The listing builds one solid part. Answer for the finished solid, in the listing's coordinates (mm). Give positions to 0.01 mm unless a question says otherwise; leave off trailing zeros. Loops run counter-clockwise (first coordinate to the right, second up) from the corner with the lowest first, then second, coordinate; pieces in that order, holes last. Notation, with made-up numbers: M -26,-33 L 15,-33 A15 cw 15,-16 Z; hole C 35,38 d7. An arc over 180 degrees is marked long. One line per item, written item: value. Start each with the question number.
Q1. A cutting plane is placed at C-C, the plane z = 36. Determine the outline of the cut face in (x, y).
Q2. A cutting plane is placed at B-B, the plane y = -5. Determine the outline of the cut face in (x, z), and give its area (3 significant figures).
Q3. A cutting plane is placed at D-D, the plane y = 39.5. Determine the outline of the cut face in (x, z).
Q4. Consider L1, parallel to Y at x = 1.3, z = 9; L2, parallel to Y at x = 0.4, z = 4; L3, parallel to Z at x = -2.15, y = 33. Determine where each line is inside the solid, lowest interval first.
Q5. A cutting plane is placed at A-A, the plane z = 4. Determine the outline of the cut face in (x, y).
from build123d import *

# Parameters (mm, degrees)
SKETCH1_R                = 59
EXTRUDE1_DEPTH           = 3
EXTRUDE2_DEPTH           = 3
CIRPATTERN1_COUNT        = 6
F_2_0_2_DIAMETER_HOLE1_D = 2
F_2_0_2_DIAMETER_HOLE3_D = 2
F_2_0_2_DIAMETER_HOLE4_D = 2
CIRPATTERN2_COUNT        = 6
CIRPATTERN3_COUNT        = 4
CIRPATTERN3_ANGLE        = 180


with BuildPart() as part:
    # Sketch1 → Extrude1 (new, symmetric)
    with BuildSketch(Plane(origin=(0, 0, 0), x_dir=(0, 0, -1), z_dir=(1, 0, 0))):
        Circle(SKETCH1_R)
        Polygon((27.939644545, 7.486405193), (7.486405193, 27.939644545), (-20.453239352, 20.453239352), (-27.939644545, -7.486405193), (-7.486405193, -27.939644545), (20.453239352, -20.453239352), align=None, mode=Mode.SUBTRACT)
    extrude(amount=EXTRUDE1_DEPTH, both=True)

    # Sketch2 → Extrude2 (add, symmetric)
    with BuildSketch(Plane(origin=(0, 0, 0), x_dir=(0, 0, -1), z_dir=(1, 0, 0))):
        with BuildLine():
            Line((-2, 67.961805723), (-0.262709442, 61.478149092))
            ThreePointArc((-0.262709442, 61.478149092), (-0.58620663, 59.77173183), (-2.122608272, 58.961805723))
            ThreePointArc((-2.122608272, 58.961805723), (28.679663449, 51.560419941), (51.21368579, 29.294340542))
            ThreePointArc((51.21368579, 29.294340542), (36.791707484, 48.186627241), (17.927108603, 62.644803614))
            ThreePointArc((17.927108603, 62.644803614), (8.312130826, 66.609702921), (-2, 67.961805723))
        make_face()
    extrude2 = extrude(amount=EXTRUDE2_DEPTH, both=True)

    # CirPattern1: Extrude2 ×6 about axis
    cirpattern1_axis = Axis((0, 0, 0), (1, 0, 0))
    for i in range(1, CIRPATTERN1_COUNT):
        add(extrude2.rotate(cirpattern1_axis, i * 360 / CIRPATTERN1_COUNT))

    # Ø2.0 (2) Diameter Hole1 (through all)
    with Locations(Plane(origin=(3, 0, 0), x_dir=(0, 0, -1), z_dir=(1, 0, 0))):
        with Locations((7.486405193, 27.939644545), (27.939644545, 7.486405193), (20.453239352, -20.453239352), (-7.486405193, -27.939644545), (-27.939644545, -7.486405193), (-20.453239352, 20.453239352)):
            Hole(F_2_0_2_DIAMETER_HOLE1_D / 2)

    # Ø2.0 (2) Diameter Hole3 (through all)
    with Locations(Plane(origin=(3, 0, 0), x_dir=(0, 0, -1), z_dir=(1, 0, 0))):
        with Locations((14.539853904, 20.886195834)):
            f_2_0_2_diameter_hole3 = Hole(F_2_0_2_DIAMETER_HOLE3_D / 2)

    # Ø2.0 (2) Diameter Hole4 (through all)
    with Locations(Plane(origin=(3, 0, 0), x_dir=(0, 0, -1), z_dir=(1, 0, 0))):
        with Locations((21.239749224, 14.186300513)):
            f_2_0_2_diameter_hole4 = Hole(F_2_0_2_DIAMETER_HOLE4_D / 2)

    # CirPattern2: Ø2.0 (2) Diameter Hole3 ×6 about axis
    cirpattern2_axis = Axis((0, 0, 0), (1, 0, 0))
    for i in range(1, CIRPATTERN2_COUNT):
        add(f_2_0_2_diameter_hole3.rotate(cirpattern2_axis, i * 360 / CIRPATTERN2_COUNT), mode=Mode.SUBTRACT)

    # CirPattern3: Ø2.0 (2) Diameter Hole4 ×4 about axis
    cirpattern3_axis = Axis((0, 0, 0), (-1, 0, 0))
    for i in range(1, CIRPATTERN3_COUNT):
        add(f_2_0_2_diameter_hole4.rotate(cirpattern3_axis, i * CIRPATTERN3_ANGLE / (CIRPATTERN3_COUNT - 1)), mode=Mode.SUBTRACT)


solid = part.part
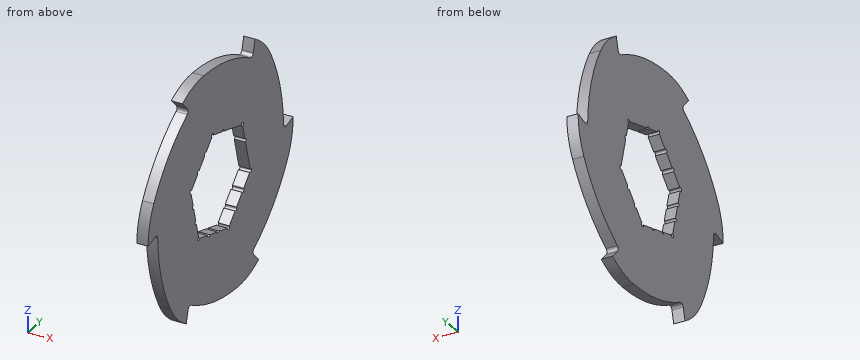
Answer block:
1. outline: M -3,-48.97 L 3,-48.97 L 3,51.54 L -3,51.54 Z
2. outline: M -3,-60.82 L 3,-60.82 L 3,-24.59 L -3,-24.59 Z; M -3,27.27 L 3,27.27 L 3,62.59 L -3,62.59 Z
2. area: 429 mm^2
3. outline: M -3,-44.41 L 3,-44.41 L 3,54.5 L -3,54.5 Z
4. L1: -66.42 to -26.43, 23.52 to 58.56
4. L2: -67.51 to -27.01, 24.86 to 58.92
4. L3: -59.29 to -55.14, -48.97 to 59.41
5. outline: M -3,-67.51 L 3,-67.51 L 3,-27.01 L -3,-27.01 Z; M -3,24.86 L 3,24.86 L 3,58.92 L -3,58.92 Z
